For this review, take the finished solid that the model builds, in its own axes (mm). Coordinates: 2 decimals unless noted, no trailing zeros. Order: outer loops, then holes, each group sorted by start corner. A loop starts at its lowest first (then second) coordinate and runs counter-clockwise, first axis right, second up. Notation, with made-up numbers: (36, 37.5) - (46, 37.5) arc R17 cw to (46, 60.5) - close; hole circle Ø4 at (40.25, 83.25). An arc over 180 degrees is marked (long way). One line per item, written item: value. Start each with the question number.
(1) Consider section C-C on z = 3.65. Count the separate pieces of the cut face and the enclosed holes in it, then the cut area to 3 significant figures.
(2) To check wall thickness, follow line 1 along Y through (x, z) = (-149, 1.25); line 2 along Y through (x, z) = (150.5, 4.6); line 3 along X through (y, z) = (5.5, 1.2). State the ranges of each line that lie inside material, in increasing order.
(3) Consider section B-B on x = -85.5. Write out the cut boundary in (y, z), then the cut area to 3 significant figures.
(4) Consider section A-A on y = -6.5. Write out the cut boundary in (x, z).
(5) Clearance check with a flat-ended pin moving along its axis: pin 1 (23 mm diameter, centred on x = -13.72, y = 2.96, fed in from -Z). State where the tip first meets the part, or that it passes through.
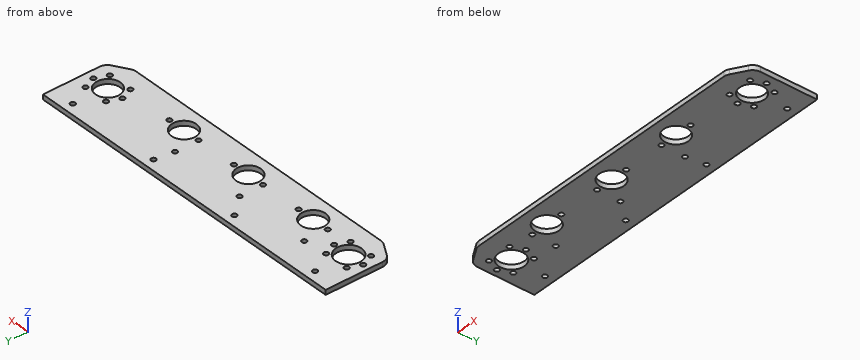
```python
from build123d import *

# Parameters (mm, degrees)
SKETCH_1_R      = 2.5
SKETCH_1_R_2    = 12.875
SKETCH_1_R_3    = 13.5
EXTRUDE_1_DEPTH = 5


with BuildPart() as part:
    # 草圖1 → 填料-伸長1 (new body)
    with BuildSketch(Plane.XY):
        with BuildLine():
            Line((-174, 57.428011653), (176, 57.428011653))
            Line((176, 57.428011653), (176, 7.612503487))
            Line((176, 7.612503487), (176, -1.381476285))
            ThreePointArc((176, -1.381476285), (174.702583739, -6.307431651), (171.146992746, -9.955184098))
            Line((171.146992746, -9.955184098), (157.274783453, -18.282988376))
            ThreePointArc((157.274783453, -18.282988376), (154.798270239, -19.346112982), (152.127790707, -19.709280563))
            Line((152.127790707, -19.709280563), (-150.840267353, -19.709280563))
            ThreePointArc((-150.840267353, -19.709280563), (-153.474646249, -19.356044157), (-155.922913438, -18.32129013))
            Line((-155.922913438, -18.32129013), (-169.082646085, -10.55466341))
            ThreePointArc((-169.082646085, -10.55466341), (-172.684079135, -6.901158615), (-174, -1.942653843))
            Line((-174, -1.942653843), (-174, 0.523128234))
            Line((-174, 0.523128234), (-174, 7.612503487))
            Line((-174, 7.612503487), (-174, 57.428011653))
        make_face()
        with Locations((131, 12.428011653)):
            Circle(SKETCH_1_R, mode=Mode.SUBTRACT)
        with Locations((167, 12.428011653)):
            Circle(SKETCH_1_R, mode=Mode.SUBTRACT)
        with Locations((149, 12.428011653)):
            Circle(SKETCH_1_R_2, mode=Mode.SUBTRACT)
        with Locations((-149, 12.428011653)):
            Circle(SKETCH_1_R_3, mode=Mode.SUBTRACT)
        with Locations((-136.272077939, 25.155933714)):
            Circle(SKETCH_1_R, mode=Mode.SUBTRACT)
        with Locations((-161.727922061, 25.155933714)):
            Circle(SKETCH_1_R, mode=Mode.SUBTRACT)
        with Locations((-136.272077939, -0.299910409)):
            Circle(SKETCH_1_R, mode=Mode.SUBTRACT)
        with Locations((-161.727922061, -0.299910409)):
            Circle(SKETCH_1_R, mode=Mode.SUBTRACT)
        with Locations((-111.854812337, 27.428011653)):
            Circle(SKETCH_1_R, mode=Mode.SUBTRACT)
        with Locations((-31.854812337, 27.428011653)):
            Circle(SKETCH_1_R, mode=Mode.SUBTRACT)
        with Locations((48.145187663, 27.428011653)):
            Circle(SKETCH_1_R, mode=Mode.SUBTRACT)
        with Locations((-93.857391311, 2.88519493)):
            Circle(SKETCH_1_R_2, mode=Mode.SUBTRACT)
        with Locations((-75.857391311, 2.88519493)):
            Circle(SKETCH_1_R, mode=Mode.SUBTRACT)
        with Locations((-111.857391311, 2.88519493)):
            Circle(SKETCH_1_R, mode=Mode.SUBTRACT)
        with Locations((-31.716358152, 2.955487842)):
            Circle(SKETCH_1_R, mode=Mode.SUBTRACT)
        with Locations((-13.716358152, 2.955487842)):
            Circle(SKETCH_1_R_2, mode=Mode.SUBTRACT)
        with Locations((4.283641848, 2.955487842)):
            Circle(SKETCH_1_R, mode=Mode.SUBTRACT)
        with Locations((48.158653697, 2.877678962)):
            Circle(SKETCH_1_R, mode=Mode.SUBTRACT)
        with Locations((66.158653697, 2.877678962)):
            Circle(SKETCH_1_R_2, mode=Mode.SUBTRACT)
        with Locations((84.158653697, 2.877678962)):
            Circle(SKETCH_1_R, mode=Mode.SUBTRACT)
        with Locations((-149, 47.428011653)):
            Circle(SKETCH_1_R, mode=Mode.SUBTRACT)
        with Locations((-49, 47.428011653)):
            Circle(SKETCH_1_R, mode=Mode.SUBTRACT)
        with Locations((51, 47.428011653)):
            Circle(SKETCH_1_R, mode=Mode.SUBTRACT)
        with Locations((151, 47.428011653)):
            Circle(SKETCH_1_R, mode=Mode.SUBTRACT)
        with Locations((-167, 12.428011653)):
            Circle(SKETCH_1_R, mode=Mode.SUBTRACT)
        with Locations((-131, 12.428011653)):
            Circle(SKETCH_1_R, mode=Mode.SUBTRACT)
        with Locations((161.727922061, -0.299910409)):
            Circle(SKETCH_1_R, mode=Mode.SUBTRACT)
        with Locations((136.272077939, -0.299910409)):
            Circle(SKETCH_1_R, mode=Mode.SUBTRACT)
        with Locations((136.272077939, 25.155933714)):
            Circle(SKETCH_1_R, mode=Mode.SUBTRACT)
        with Locations((161.727922061, 25.155933714)):
            Circle(SKETCH_1_R, mode=Mode.SUBTRACT)
    extrude(amount=EXTRUDE_1_DEPTH)


solid = part.part
```
Geometry check:
1. separate pieces: 1
1. enclosed holes: 30
1. area: 23,600 mm^2
2. line 1: y = -19.71 to -1.07, 25.93 to 44.93, 49.93 to 57.43
2. line 2: y = -19.71 to -0.36, 25.22 to 44.98, 49.88 to 57.43
2. line 3: x = -174 to -160.59, -137.41 to -106.46, -81.25 to -26.34, -1.1 to 53.55, 78.76 to 138.15, 159.85 to 176
3. outline: (-19.71, 0) - (-6.91, 0) - (-6.91, 5) - (-19.71, 5) - close; (12.68, 0) - (57.43, 0) - (57.43, 5) - (12.68, 5) - close
3. area: 288 mm^2
4. outline: (-172.9, 0) - (-102.67, 0) - (-102.67, 5) - (-172.9, 5) - close; (-85.04, 0) - (-22.45, 0) - (-22.45, 5) - (-85.04, 5) - close; (-4.98, 0) - (57.34, 0) - (57.34, 5) - (-4.98, 5) - close; (74.98, 0) - (174.59, 0) - (174.59, 5) - (74.98, 5) - close
5. pin 1: passes through
